from build123d import *

# Parameters (mm, degrees)
F0_W      = 3
F0_H      = 3
F1_DEPTH  = 35
F2_R      = 2
F3_DEPTH  = 3
F4_R      = 2
F5_DEPTH  = 3
F6_R      = 2
F7_DEPTH  = 3
F8_R      = 2
F9_DEPTH  = 3
F10_R     = 2
F11_DEPTH = 3
F12_R     = 2
F13_DEPTH = 3


with BuildPart() as f1:
    # F0 (on Front) → F1 (new body, symmetric)
    with BuildSketch(Plane.XZ):
        Polygon((-35, 35), (-35, 32), (-32, 32), (-14, 32), (14, 32), (32, 32), (32, 35), align=None)
        Polygon((35, 32), (32, 32), (32, 14), (32, -14), (32, -32), (35, -32), (35, 0), align=None)
        with Locations((33.5, 33.5)):
            Rectangle(F0_W, F0_H)
        Polygon((-35, 32), (-35, 0), (-35, -32), (-32, -32), (-32, -14), (-32, 14), (-32, 32), align=None)
        Polygon((-14, -32), (-32, -32), (-32, -35), (32, -35), (32, -32), (14, -32), align=None)
        with Locations((-33.5, -33.5)):
            Rectangle(F0_W, F0_H)
        with Locations((33.5, -33.5)):
            Rectangle(F0_W, F0_H)
    extrude(amount=F1_DEPTH, both=True)

    # F2 (on face) → F3 (join)
    with BuildSketch(Plane.XZ.offset(35)):
        with BuildLine():
            Line((-32, 14), (-18, 14))
            ThreePointArc((-18, 14), (-20.8284271247, 20.8284271247), (-14, 18))
            Line((-14, 18), (-14, 32))
            Line((-14, 32), (-32, 32))
            Line((-32, 32), (-32, 14))
        make_face()
        with BuildLine():
            ThreePointArc((-14, 18), (-20.8284271247, 20.8284271247), (-18, 14))
            ThreePointArc((-18, 14), (-15.1715728753, 15.1715728753), (-14, 18))
        make_face()
        with Locations((-18, 18)):
            Circle(F2_R, mode=Mode.SUBTRACT)
        with BuildLine():
            ThreePointArc((22, 18), (18, 22), (14, 18))
            ThreePointArc((14, 18), (15.1715728753, 15.1715728753), (18, 14))
            ThreePointArc((18, 14), (20.8284271247, 15.1715728753), (22, 18))
        make_face()
        with Locations((18, 18)):
            Circle(F2_R, mode=Mode.SUBTRACT)
        with BuildLine():
            Line((32, 32), (14, 32))
            Line((14, 32), (14, 18))
            ThreePointArc((14, 18), (18, 22), (22, 18))
            ThreePointArc((22, 18), (20.8284271247, 15.1715728753), (18, 14))
            Line((18, 14), (32, 14))
            Line((32, 14), (32, 32))
        make_face()
        with BuildLine():
            Line((14, -18), (14, -32))
            Line((14, -32), (32, -32))
            Line((32, -32), (32, -14))
            Line((32, -14), (18, -14))
            ThreePointArc((18, -14), (20.8284271247, -15.1715728753), (22, -18))
            ThreePointArc((22, -18), (18, -22), (14, -18))
        make_face()
        with BuildLine():
            ThreePointArc((18, -14), (15.1715728753, -15.1715728753), (14, -18))
            ThreePointArc((14, -18), (18, -22), (22, -18))
            ThreePointArc((22, -18), (20.8284271247, -15.1715728753), (18, -14))
        make_face()
        with Locations((18, -18)):
            Circle(F2_R, mode=Mode.SUBTRACT)
        with BuildLine():
            ThreePointArc((-14, -18), (-15.1715728753, -15.1715728753), (-18, -14))
            ThreePointArc((-18, -14), (-20.8284271247, -20.8284271247), (-14, -18))
        make_face()
        with Locations((-18, -18)):
            Circle(F2_R, mode=Mode.SUBTRACT)
        with BuildLine():
            Line((-18, -14), (-32, -14))
            Line((-32, -14), (-32, -32))
            Line((-32, -32), (-14, -32))
            Line((-14, -32), (-14, -18))
            ThreePointArc((-14, -18), (-20.8284271247, -20.8284271247), (-18, -14))
        make_face()
    extrude(amount=-F3_DEPTH)

    # F4 (on face) → F5 (join)
    with BuildSketch(Plane(origin=(0, 35, 0), x_dir=(-1, 0, 0), z_dir=(0, 1, 0))):
        with BuildLine():
            Line((-14, 18), (-14, 32))
            Line((-14, 32), (-32, 32))
            Line((-32, 32), (-32, 14))
            Line((-32, 14), (-18, 14))
            ThreePointArc((-18, 14), (-20.8284271247, 20.8284271247), (-14, 18))
        make_face()
        with BuildLine():
            ThreePointArc((-18, 14), (-15.1715728753, 15.1715728753), (-14, 18))
            ThreePointArc((-14, 18), (-20.8284271247, 20.8284271247), (-18, 14))
        make_face()
        with Locations((-18, 18)):
            Circle(F4_R, mode=Mode.SUBTRACT)
        with BuildLine():
            Line((14, 32), (14, 18))
            ThreePointArc((14, 18), (18, 22), (22, 18))
            ThreePointArc((22, 18), (20.8284271247, 15.1715728753), (18, 14))
            Line((18, 14), (32, 14))
            Line((32, 14), (32, 32))
            Line((32, 32), (14, 32))
        make_face()
        with BuildLine():
            ThreePointArc((22, 18), (18, 22), (14, 18))
            ThreePointArc((14, 18), (15.1715728753, 15.1715728753), (18, 14))
            ThreePointArc((18, 14), (20.8284271247, 15.1715728753), (22, 18))
        make_face()
        with Locations((18, 18)):
            Circle(F4_R, mode=Mode.SUBTRACT)
        with BuildLine():
            Line((32, -32), (32, -14))
            Line((32, -14), (18, -14))
            ThreePointArc((18, -14), (20.8284271247, -15.1715728753), (22, -18))
            ThreePointArc((22, -18), (18, -22), (14, -18))
            Line((14, -18), (14, -32))
            Line((14, -32), (32, -32))
        make_face()
        with BuildLine():
            ThreePointArc((22, -18), (20.8284271247, -15.1715728753), (18, -14))
            ThreePointArc((18, -14), (15.1715728753, -15.1715728753), (14, -18))
            ThreePointArc((14, -18), (18, -22), (22, -18))
        make_face()
        with Locations((18, -18)):
            Circle(F4_R, mode=Mode.SUBTRACT)
        with BuildLine():
            ThreePointArc((-14, -18), (-15.1715728753, -15.1715728753), (-18, -14))
            ThreePointArc((-18, -14), (-20.8284271247, -20.8284271247), (-14, -18))
        make_face()
        with Locations((-18, -18)):
            Circle(F4_R, mode=Mode.SUBTRACT)
        with BuildLine():
            Line((-18, -14), (-32, -14))
            Line((-32, -14), (-32, -32))
            Line((-32, -32), (-14, -32))
            Line((-14, -32), (-14, -18))
            ThreePointArc((-14, -18), (-20.8284271247, -20.8284271247), (-18, -14))
        make_face()
    extrude(amount=-F5_DEPTH)

    # F6 (on face) → F7 (cut)
    with BuildSketch(Plane.YZ.offset(35)):
        with BuildLine():
            Line((14, 32), (-14, 32))
            Line((-14, 32), (-14, 18))
            ThreePointArc((-14, 18), (-15.1715728753, 15.1715728753), (-18, 14))
            Line((-18, 14), (-32, 14))
            Line((-32, 14), (-32, -14))
            Line((-32, -14), (-18, -14))
            ThreePointArc((-18, -14), (-15.1715728753, -15.1715728753), (-14, -18))
            Line((-14, -18), (-14, -32))
            Line((-14, -32), (14, -32))
            Line((14, -32), (14, -18))
            ThreePointArc((14, -18), (15.1715728753, -15.1715728753), (18, -14))
            Line((18, -14), (32, -14))
            Line((32, -14), (32, 14))
            Line((32, 14), (18, 14))
            ThreePointArc((18, 14), (15.1715728753, 15.1715728753), (14, 18))
            Line((14, 18), (14, 32))
        make_face()
        with Locations((-18, 18)):
            Circle(F6_R)
        with Locations((18, 18)):
            Circle(F6_R)
        with Locations((18, -18)):
            Circle(F6_R)
        with Locations((-18, -18)):
            Circle(F6_R)
    extrude(amount=-F7_DEPTH, mode=Mode.SUBTRACT)

    # F8 (on face) → F9 (cut)
    with BuildSketch(Plane(origin=(-35, 0, 0), x_dir=(0, -1, 0), z_dir=(-1, 0, 0))):
        with BuildLine():
            ThreePointArc((-14, 18), (-15.1715728753, 15.1715728753), (-18, 14))
            Line((-18, 14), (-32, 14))
            Line((-32, 14), (-32, -14))
            Line((-32, -14), (-18, -14))
            ThreePointArc((-18, -14), (-15.1715728753, -15.1715728753), (-14, -18))
            Line((-14, -18), (-14, -32))
            Line((-14, -32), (14, -32))
            Line((14, -32), (14, -18))
            ThreePointArc((14, -18), (15.1715728753, -15.1715728753), (18, -14))
            Line((18, -14), (32, -14))
            Line((32, -14), (32, 14))
            Line((32, 14), (18, 14))
            ThreePointArc((18, 14), (15.1715728753, 15.1715728753), (14, 18))
            Line((14, 18), (14, 32))
            Line((14, 32), (-14, 32))
            Line((-14, 32), (-14, 18))
        make_face()
        with Locations((-18, 18)):
            Circle(F8_R)
        with Locations((18, 18)):
            Circle(F8_R)
        with Locations((18, -18)):
            Circle(F8_R)
        with Locations((-18, -18)):
            Circle(F8_R)
    extrude(amount=-F9_DEPTH, mode=Mode.SUBTRACT)

    # F10 (on face) → F11 (cut)
    with BuildSketch(Plane.XY.offset(35)):
        with BuildLine():
            Line((14, 32), (-14, 32))
            Line((-14, 32), (-14, 18))
            ThreePointArc((-14, 18), (-15.1715728753, 15.1715728753), (-18, 14))
            Line((-18, 14), (-32, 14))
            Line((-32, 14), (-32, -14))
            Line((-32, -14), (-18, -14))
            ThreePointArc((-18, -14), (-15.1715728753, -15.1715728753), (-14, -18))
            Line((-14, -18), (-14, -32))
            Line((-14, -32), (14, -32))
            Line((14, -32), (14, -18))
            ThreePointArc((14, -18), (15.1715728753, -15.1715728753), (18, -14))
            Line((18, -14), (32, -14))
            Line((32, -14), (32, 14))
            Line((32, 14), (18, 14))
            ThreePointArc((18, 14), (15.1715728753, 15.1715728753), (14, 18))
            Line((14, 18), (14, 32))
        make_face()
        with Locations((-18, 18)):
            Circle(F10_R)
        with Locations((18, 18)):
            Circle(F10_R)
        with Locations((18, -18)):
            Circle(F10_R)
        with Locations((-18, -18)):
            Circle(F10_R)
    extrude(amount=-F11_DEPTH, mode=Mode.SUBTRACT)

    # F12 (on face) → F13 (cut)
    with BuildSketch(Plane(origin=(0, 0, -35), x_dir=(1, 0, 0), z_dir=(0, 0, -1))):
        with BuildLine():
            Line((14, 32), (-14, 32))
            Line((-14, 32), (-14, 18))
            ThreePointArc((-14, 18), (-15.1715728753, 15.1715728753), (-18, 14))
            Line((-18, 14), (-32, 14))
            Line((-32, 14), (-32, -14))
            Line((-32, -14), (-18, -14))
            ThreePointArc((-18, -14), (-15.1715728753, -15.1715728753), (-14, -18))
            Line((-14, -18), (-14, -32))
            Line((-14, -32), (14, -32))
            Line((14, -32), (14, -18))
            ThreePointArc((14, -18), (15.1715728753, -15.1715728753), (18, -14))
            Line((18, -14), (32, -14))
            Line((32, -14), (32, 14))
            Line((32, 14), (18, 14))
            ThreePointArc((18, 14), (15.1715728753, 15.1715728753), (14, 18))
            Line((14, 18), (14, 32))
        make_face()
        with Locations((-18, 18)):
            Circle(F12_R)
        with Locations((-18, -18)):
            Circle(F12_R)
        with Locations((18, -18)):
            Circle(F12_R)
        with Locations((18, 18)):
            Circle(F12_R)
    extrude(amount=-F13_DEPTH, mode=Mode.SUBTRACT)


solid = f1.part
Input: part model. Units: mm. Frame: model coordinates. A direction names the side the tool comes from. Give positions to 0.01 mm unless a question says otherwise; leave off trailing zeros. Order: outer loops, then holes, each group sorted by start corner. A loop starts at its lowest first (then second) coordinate and runs counter-clockwise, first axis right, second up. Notation, with made-up numbers: M 7.25,88.5 L 55.25,88.5 A12 cw 55.25,105.5 Z; hole C 29.5,32.5 d2. An arc over 180 degrees is marked long. Answer as a JSON object with one key per item and string values.
1. Cut plane C-C, the plane z = 5.5. Output: boundary loops of the cut face in (x, y).
Result sheet:
{"outline": "M -35,-35 L -32,-35 L -32,-32 L -35,-32 Z; M -35,32 L -32,32 L -32,35 L -35,35 Z; M 32,-35 L 35,-35 L 35,-32 L 32,-32 Z; M 32,32 L 35,32 L 35,35 L 32,35 Z"}
2. Pull-direction query (X, two-part tool) for faces 5 (the flat face through (34, 25, 14)), 6 (the flat face through (-23, 32, -23)), 7 (the flat face through (-25, 14, -34)); classes: +X half, -X half, draft (parallel to the pull), parting line (faces both ways), or undercut.
Result sheet:
{"face 5": "draft", "face 6": "undercut", "face 7": "undercut"}
3. Cut plane A-A, the plane y = -23. Output: boundary loops of the cut face in (x, z), and give its area (3 significant figures).
Result sheet:
{"outline": "M -35,-35 L -14,-35 L -14,-32 L -32,-32 L -32,-14 L -35,-14 Z; M -35,14 L -32,14 L -32,32 L -14,32 L -14,35 L -35,35 Z; M 14,-35 L 35,-35 L 35,-14 L 32,-14 L 32,-32 L 14,-32 Z; M 14,32 L 32,32 L 32,14 L 35,14 L 35,35 L 14,35 Z", "area": "468 mm²"}
4. First-contact query: P1, Ø12, axis at x = -5.5, y = 28, coming from the +Z side; P2, Ø3.5, axis at x = -18, y = 18, coming from the -Z side. Flat tips, straight axial feed; report the tip coordinate or a pass-through.
Result sheet:
{"P1": "z = 35", "P2": "through"}
5. Reachability of faces 1 (the cylindrical face through (-33.521, 15.141, 15.203)), 2 (the flat face through (-25, 34, -14)), 3 (the flat face through (25, 14, -34)), 4 (the flat face through (23, -32, 23)) from +Z, -Z, +X, -X, +Y, -Y: full face, straight path, thin tool, end or side. Return the list, or none.
Result sheet:
{"face 1": "+X, -X", "face 2": "+Y, -Y", "face 3": "+Z, -Z", "face 4": "none"}
6. Ray query, line 1 (Y direction, x = 14.5, z = 26.5). Return the intervals inside material, ascending. Write a range as [from, to].
Result sheet:
{"line 1": "[-35, -32], [32, 35]"}
